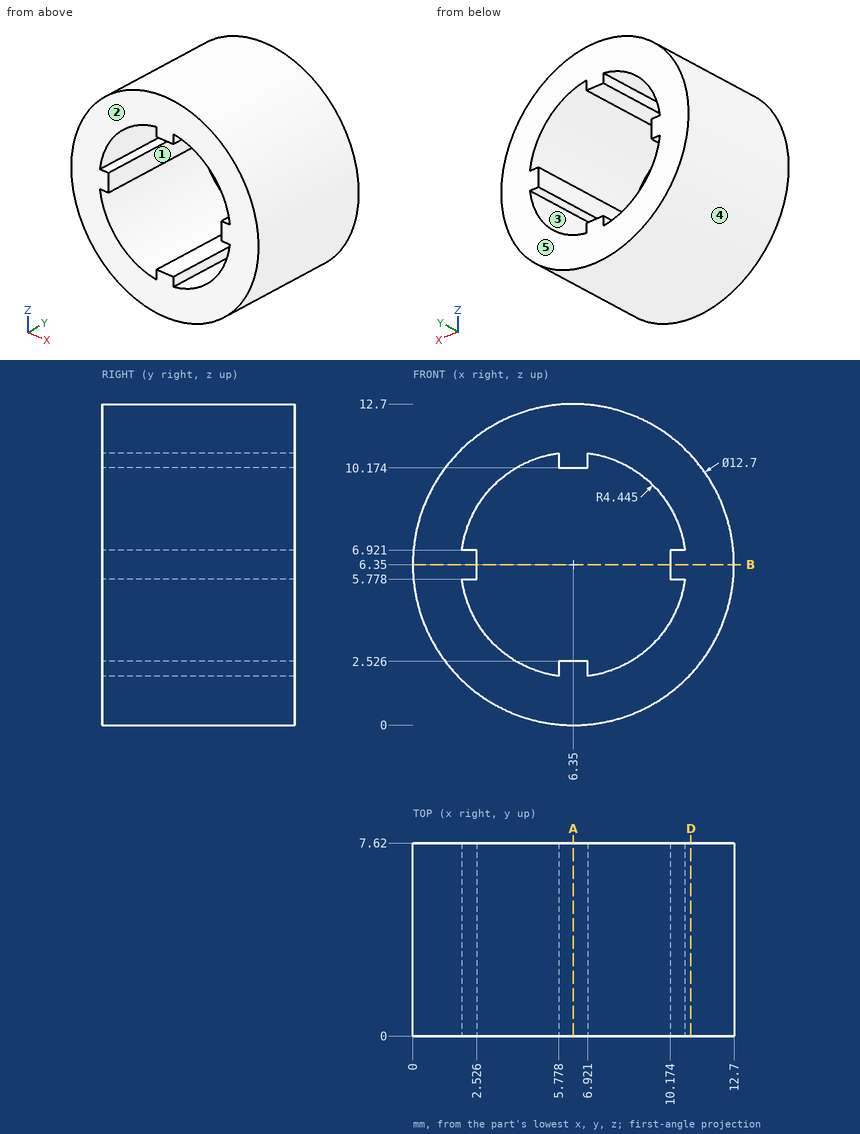
Geometry: see drawing. Coordinates: mm, zero at the bounding-box minimum. A direction names the side the tool comes from. Round coordinates to 2 decimals unless told otherwise and drop trailing zeros. Loops run counter-clockwise (first coordinate to the right, second up) from the corner with the lowest first, then second, coordinate; pieces in that order, holes last. Notation, with made-up numbers: (41.5, -9.5) -> (47.5, -9.5) arc R24 ccw to (47.5, 29.5) -> close; hole circle Ø8 at (62, 51.25). An arc over 180 degrees is marked (long way). Write each question's results on one line, items separated by ' | '.
Item 1: Line query: probe 1 along X at (y, z) = (4.25, 6.25); probe 2 along Z at (x, y) = (4.5, 5.5) (1 decimal); probe 3 along X at (y, z) = (4.5, 7.25) (1 decimal). Output: solid intervals per line, ascending. Write a range as [from, to].
Answers below:
probe 1: x = [0, 2.53], [10.17, 12.7] | probe 2: z = [0.3, 2.3], [10.4, 12.4] | probe 3: x = [0.1, 2], [10.7, 12.6]
Item 2: Pin query (flat end, axial travel): pin 1 Ø0.6 at (y, z) = (4.5, 2.5) entering from -X (1 decimal); pin 2 Ø2 at (x, y) = (3.5, 2) entering from +Z (1 decimal); pin 3 Ø1.5 at (x, z) = (3.5, 4.5) entering from +Y; pin 4 Ø0.5 at (x, y) = (10.5, 3) entering from -Z. Return the tip coordinate at first contact, or that it passes through.
Answers below:
pin 1: stops at x = 1.1 | pin 2: stops at z = 12.4 | pin 3: passes through | pin 4: stops at z = 1.34
Item 3: Pull-direction query (X, two-part tool) for the marked faces 3, 4 and 5; classes: pulls with the +X half, pulls with the -X half, needs draft (parallel to the pull), parting line crosses it, or undercut.
Answers below:
face 3: undercut | face 4: parting line crosses it | face 5: needs draft
Item 4: Cut plane B-B on z = 6.35. Return the cut outline in (x, y), and give its area (3 significant figures).
Answers below:
outline: (0, 0) -> (2.53, 0) -> (2.53, 7.62) -> (0, 7.62) -> close; (10.17, 0) -> (12.7, 0) -> (12.7, 7.62) -> (10.17, 7.62) -> close | area: 38.5 mm²
Item 5: Set-up query: the marked faces 1 and 2. Return all of +Z, -Z, +X, -X, +Y, -Y with unobstructed straight access to the full face (end or side cutting, diameter ignored); none if empty.
Answers below:
face 1: +Y, -Y | face 2: +Z, -Z, +X, -X, -Y
Item 6: Cut plane A-A on x = 6.35. Return the cut outline in (y, z), and give its area (3 significant figures).
Answers below:
outline: (0, 0) -> (7.62, 0) -> (7.62, 2.53) -> (0, 2.53) -> close; (0, 10.17) -> (7.62, 10.17) -> (7.62, 12.7) -> (0, 12.7) -> close | area: 38.5 mm²
Item 7: Cut plane D-D on x = 11. Return the cut outline in (y, z) (1 decimal).
Answers below:
outline: (0, 2) -> (7.6, 2) -> (7.6, 10.7) -> (0, 10.7) -> close
